The model under review builds one solid part; all positions refer to its coordinate system, in mm. A direction names the side the tool comes from. Coordinates: 2 decimals unless noted, no trailing zeros. Order: outer loops, then holes, each group sorted by start corner. A loop starts at its lowest first (then second) coordinate and runs counter-clockwise, first axis right, second up. Notation, with made-up numbers: (70, 48.5) -> (96, 48.5) arc R20 cw to (96, 60.5) -> close; hole circle Ø3 at (11, -3). An arc over 180 degrees is marked (long way). Use one line per item in the form item = value. Start each with the question number.
(1) Mouldability with a two-part tool opening along X and no side actions: class faces 3 (the cylindrical face through (15.272, 17.235, 1.479)), 4 (the flat face through (20, 0, 1)), 5 (the cylindrical face through (-19, -18, 1)) as +X half, -X half, draft (parallel to the pull), parting line (faces both ways), or undercut.
(2) Insertion check: pin 1 Ø5 at (y, z) = (-8, 7.5) entering from -X; pin 2 Ø4 at (x, y) = (15.5, 15.5) entering from +Z; pin 3 Ø1.5 at (y, z) = (-8.5, 5.5) entering from +X. Each pin has a flat end and moves straight along its axis. Give the tip position at first contact, or say it passes through.
(3) Take a section at A-A (x = 0). State the section outline as (y, z) points, then the cut area to 3 significant figures.
(4) For faces 1 (the cylindrical face through (5.19, -9.98, 6.45)), 2 (the cylindrical face through (-14.6, -14, 1.5)), list the 3-axis set-ups (+Z, -Z, +X, -X, +Y, -Y) from which the entire face can be reached by the end or side of a thin tool; tool diameter is ignored.
(5) Take a section at C-C (z = 1). State the section outline as (x, y) points.
(6) Take a section at D-D (z = 9.25). State the section outline as (x, y) points, then the cut area to 3 significant figures.
(7) Wall thickness on line 1 along X through (y, z) = (-15.5, 1.7); line 2 along X through (y, z) = (0, 1.65): over which ranges is each line inside the solid? List them lowest first.
```python
from build123d import *

# Parameters (mm, degrees)
CYLINDER001_R     = 11.25
CYLINDER001_DEPTH = 7
CYLINDER_R        = 13
CYLINDER_DEPTH    = 7
SKETCH_R          = 1.75
SKETCH_R_2        = 4.5
PAD_DEPTH         = 4
BOX_W             = 40
BOX_H             = 40
BOX_DEPTH         = 3
CHAMFER_SIZE      = 2
FILLET_R          = 5
FILLET001_R       = 1


with BuildPart() as obj1:
    # Cylinder001 → Cylinder001 (new body)
    with BuildSketch(Plane.XY):
        Circle(CYLINDER001_R)
    extrude(amount=CYLINDER001_DEPTH)


with BuildPart() as cut001:
    # Cylinder → Cylinder (new body)
    with BuildSketch(Plane.XY):
        Circle(CYLINDER_R)
    extrude(amount=CYLINDER_DEPTH)

    # Cut001: cut obj1
    add(obj1.part, mode=Mode.SUBTRACT)


with BuildPart() as cut001_1:
    # Cut001 placement: moved
    add(cut001.part.moved(Location((0, 0, 3))))


with BuildPart() as pad:
    # Sketch → Pad (new body)
    with BuildSketch(Plane.XY.offset(-0.5)):
        with Locations((-15.5, 15.5)):
            Circle(SKETCH_R)
        with Locations((15.5, 15.5)):
            Circle(SKETCH_R)
        with Locations((-15.5, -15.5)):
            Circle(SKETCH_R)
        with Locations((15.5, -15.5)):
            Circle(SKETCH_R)
        Circle(SKETCH_R_2)
    extrude(amount=PAD_DEPTH)


with BuildPart() as x_end_idler_cnc:
    # Box → Box (new body)
    with BuildSketch(Plane(origin=(-20, -20, 0), x_dir=(1, 0, 0), z_dir=(0, 0, 1))):
        with Locations((20, 20)):
            Rectangle(BOX_W, BOX_H)
    extrude(amount=BOX_DEPTH)

    # Cut: cut Pad
    add(pad.part, mode=Mode.SUBTRACT)

    # Fusion: union Cut001
    add(cut001_1.part)

    # Chamfer
    chamfer_edges = [x_end_idler_cnc.edges().sort_by_distance(p)[0] for p in [
        (-13, 0, 3),
    ]]
    chamfer(chamfer_edges, length=CHAMFER_SIZE)

    # Fillet
    fillet_edges = [x_end_idler_cnc.edges().sort_by_distance(p)[0] for p in [
        (-20, -20, 1.5),
        (-20, 20, 1.5),
        (20, 20, 1.5),
        (20, -20, 1.5),
    ]]
    fillet(fillet_edges, radius=FILLET_R)

    # Fillet001
    fillet001_edges = [x_end_idler_cnc.edges().sort_by_distance(p)[0] for p in [
        (-20, 0, 3),
        (-18.535534, -18.535534, 3),
        (-18.535534, 18.535534, 3),
        (0, -20, 3),
        (0, 20, 3),
        (18.535534, -18.535534, 3),
        (18.535534, 18.535534, 3),
        (20, 0, 3),
    ]]
    fillet(fillet001_edges, radius=FILLET001_R)


solid = x_end_idler_cnc.part
```
Findings:
q1.face_3 = undercut
q1.face_4 = +X half
q1.face_5 = -X half
q2.pin_1 = -11.78
q2.pin_2 = 3
q2.pin_3 = 10.44
q3.outline = (-20, 0) -> (-4.5, 0) -> (-4.5, 3) -> (-11.25, 3) -> (-11.25, 10) -> (-13, 10) -> (-13, 5) -> (-15, 3) -> (-19, 3) arc R1 ccw to (-20, 2) -> close; (4.5, 0) -> (20, 0) -> (20, 2) arc R1 ccw to (19, 3) -> (15, 3) -> (13, 5) -> (13, 10) -> (11.25, 10) -> (11.25, 3) -> (4.5, 3) -> close
q3.area = 121 mm²
q4.face_1 = +Z
q4.face_2 = +Z, -Z
q5.outline = (-20, -15) arc R5 ccw to (-15, -20) -> (15, -20) arc R5 ccw to (20, -15) -> (20, 15) arc R5 ccw to (15, 20) -> (-15, 20) arc R5 ccw to (-20, 15) -> close; hole circle Ø3.5 at (-15.5, -15.5); hole circle Ø3.5 at (-15.5, 15.5); hole circle Ø9 at (0, 0); hole circle Ø3.5 at (15.5, -15.5); hole circle Ø3.5 at (15.5, 15.5)
q6.outline = circle Ø26 at (0, 0); hole circle Ø22.5 at (0, 0)
q6.area = 133 mm²
q7.line_1 = -19.97 to -17.25, -13.75 to 13.75, 17.25 to 19.97
q7.line_2 = -20 to -4.5, 4.5 to 20
